```python
from build123d import *

# Parameters (mm, degrees)
SKETCH1_W                   = 203.2
SKETCH1_H                   = 203.2
BOSS_EXTRUDE1_DEPTH         = 6.35
CUT_EXTRUDE1_REACH          = 8.35
SKETCH2_R                   = 76.2
F_1_4_20_TAPPED_HOLE1_D     = 5.1054
F_1_4_20_TAPPED_HOLE1_DEPTH = 6.351
CIRPATTERN1_COUNT           = 12
CUT_EXTRUDE2_REACH          = 8.35


with BuildPart() as part:
    # Sketch1 → Boss-Extrude1 (new body)
    with BuildSketch(Plane(origin=(0, 0, 0), x_dir=(1, 0, 0), z_dir=(0, 1, 0))):
        Rectangle(SKETCH1_W, SKETCH1_H)
    extrude(amount=BOSS_EXTRUDE1_DEPTH)

    # Sketch2 → Cut-Extrude1 (cut, up to next)
    with BuildSketch(Plane(origin=(0, 6.35, 0), x_dir=(1, 0, 0), z_dir=(0, 1, 0)), mode=Mode.PRIVATE) as cut_extrude1_sk1:
        with Locations(Location((0, 0, 0), (0, 0, 270))):  # turned: the seam where the file's is
            Circle(SKETCH2_R)
    cut_extrude1_tool1 = extrude(cut_extrude1_sk1.sketch, amount=-CUT_EXTRUDE1_REACH, mode=Mode.PRIVATE) & part.part
    add(cut_extrude1_tool1.solids().sort_by_distance((0, 6.35, 0))[0], mode=Mode.SUBTRACT)

    # 1/4-20 Tapped Hole1
    with Locations(Plane(origin=(0, 6.35, 0), x_dir=(1, 0, 0), z_dir=(0, 1, 0))):
        with Locations((0, 85.725)):
            f_1_4_20_tapped_hole1 = Hole(F_1_4_20_TAPPED_HOLE1_D / 2, depth=F_1_4_20_TAPPED_HOLE1_DEPTH)

    # CirPattern1: 1/4-20 Tapped Hole1 ×12 about axis
    cirpattern1_axis = Axis((0, 0, 0), (0, 1, 0))
    for i in range(1, CIRPATTERN1_COUNT):
        add(f_1_4_20_tapped_hole1.rotate(cirpattern1_axis, i * 360 / CIRPATTERN1_COUNT), mode=Mode.SUBTRACT)

    # Sketch5 → Cut-Extrude2 (cut, up to next)
    with BuildSketch(Plane(origin=(0, 6.35, 0), x_dir=(1, 0, 0), z_dir=(0, 1, 0)), mode=Mode.PRIVATE) as cut_extrude2_sk1:
        with BuildLine():
            ThreePointArc((-45.084916162, 96.684914721), (-75.434151417, 75.434151417), (-96.684914721, 45.084916162))
            ThreePointArc((-96.684914721, 45.084916162), (-95.149200478, 40.865575958), (-90.929860273, 42.4012902))
            ThreePointArc((-90.929860273, 42.4012902), (-70.944023356, 70.944023356), (-42.4012902, 90.929860273))
            ThreePointArc((-42.4012902, 90.929860273), (-40.865575958, 95.149200478), (-45.084916162, 96.684914721))
        make_face()
    cut_extrude2_tool1 = extrude(cut_extrude2_sk1.sketch, amount=-CUT_EXTRUDE2_REACH, mode=Mode.PRIVATE) & part.part
    add(cut_extrude2_tool1.solids().sort_by_distance((-71.522214, 6.35, -71.522214))[0], mode=Mode.SUBTRACT)
    # Sketch5 → Cut-Extrude2 (cut, up to next)
    with BuildSketch(Plane(origin=(0, 6.35, 0), x_dir=(1, 0, 0), z_dir=(0, 1, 0)), mode=Mode.PRIVATE) as cut_extrude2_sk2:
        with BuildLine():
            ThreePointArc((96.684914721, 45.084916162), (75.434151417, 75.434151417), (45.084916162, 96.684914721))
            ThreePointArc((45.084916162, 96.684914721), (40.865575958, 95.149200478), (42.4012902, 90.929860273))
            ThreePointArc((42.4012902, 90.929860273), (70.944023356, 70.944023356), (90.929860273, 42.4012902))
            ThreePointArc((90.929860273, 42.4012902), (95.149200478, 40.865575958), (96.684914721, 45.084916162))
        make_face()
    cut_extrude2_tool2 = extrude(cut_extrude2_sk2.sketch, amount=-CUT_EXTRUDE2_REACH, mode=Mode.PRIVATE) & part.part
    add(cut_extrude2_tool2.solids().sort_by_distance((71.522214, 6.35, -71.522214))[0], mode=Mode.SUBTRACT)
    # Sketch5 → Cut-Extrude2 (cut, up to next)
    with BuildSketch(Plane(origin=(0, 6.35, 0), x_dir=(1, 0, 0), z_dir=(0, 1, 0)), mode=Mode.PRIVATE) as cut_extrude2_sk3:
        with BuildLine():
            ThreePointArc((-96.684914721, -45.084916162), (-75.434151417, -75.434151417), (-45.084916162, -96.684914721))
            ThreePointArc((-45.084916162, -96.684914721), (-40.865575958, -95.149200478), (-42.4012902, -90.929860273))
            ThreePointArc((-42.4012902, -90.929860273), (-70.944023356, -70.944023356), (-90.929860273, -42.4012902))
            ThreePointArc((-90.929860273, -42.4012902), (-95.149200478, -40.865575958), (-96.684914721, -45.084916162))
        make_face()
    cut_extrude2_tool3 = extrude(cut_extrude2_sk3.sketch, amount=-CUT_EXTRUDE2_REACH, mode=Mode.PRIVATE) & part.part
    add(cut_extrude2_tool3.solids().sort_by_distance((-71.522214, 6.35, 71.522214))[0], mode=Mode.SUBTRACT)
    # Sketch5 → Cut-Extrude2 (cut, up to next)
    with BuildSketch(Plane(origin=(0, 6.35, 0), x_dir=(1, 0, 0), z_dir=(0, 1, 0)), mode=Mode.PRIVATE) as cut_extrude2_sk4:
        with BuildLine():
            ThreePointArc((45.084916162, -96.684914721), (75.434151417, -75.434151417), (96.684914721, -45.084916162))
            ThreePointArc((96.684914721, -45.084916162), (95.149200478, -40.865575958), (90.929860273, -42.4012902))
            ThreePointArc((90.929860273, -42.4012902), (70.944023356, -70.944023356), (42.4012902, -90.929860273))
            ThreePointArc((42.4012902, -90.929860273), (40.865575958, -95.149200478), (45.084916162, -96.684914721))
        make_face()
    cut_extrude2_tool4 = extrude(cut_extrude2_sk4.sketch, amount=-CUT_EXTRUDE2_REACH, mode=Mode.PRIVATE) & part.part
    add(cut_extrude2_tool4.solids().sort_by_distance((71.522214, 6.35, 71.522214))[0], mode=Mode.SUBTRACT)


solid = part.part
```
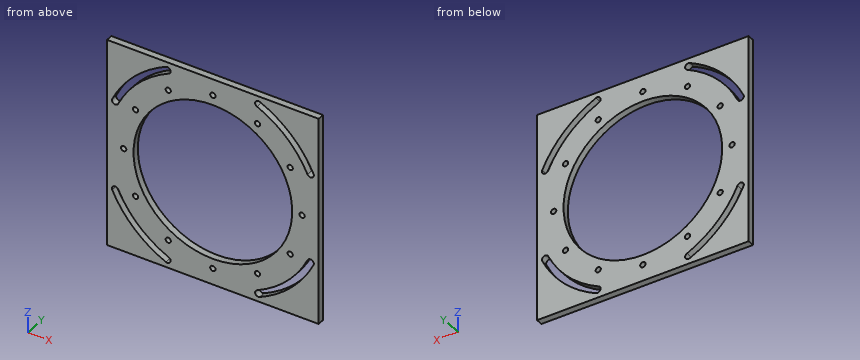
Verification items for the finished model (mm, model axes). Coordinates: 2 decimals unless noted, no trailing zeros. Write each loop counter-clockwise with the first axis right and the second up, starting at its lowest first coordinate (ties: lowest second). Pieces come first, ordered by that corner, then holes. Notation, with made-up numbers: M 36,14.25 L 82,14.25 A14 cw 82,19.25 Z; hole C 0.5,78.5 d10. An arc over 180 degrees is marked long. Answer as a JSON object with one key per item and string values. Group by question number.
(1) Cross-section at D-D, the plane y = 2.25. State how many separate pieces and enclosed holes the cut face has, and give its area (3 significant figures).
(2) Gauge pin test, flat end, axial feed: pin 1 (1 mm diameter, centred on x = -35.5, z = -66.5, fed in from -Y). Record the tip position at first contact, or that the pin passes through.
(3) Material ranges on line 1 (X direction, y = 0.5, z = -83); line 2 (Z direction, x = 56, y = 4.5); line 3 (Z direction, x = -64, y = 5), recorded low to high.
(4) Cross-section at A-A, the plane z = 0. Record the cut outline in (x, y).
(5) Cross-section at B-B, the plane x = 0. Record the cut outline in (y, z), and give its area (3 significant figures).
(6) Cross-section at C-C, the plane z = 22. Record the cut outline in (x, y).
Reply:
{
 "1": {"separate pieces": "1", "enclosed holes": "17", "area": "20,800 mm²"},
 "2": {"pin 1": "through"},
 "3": {"line 1": "-101.6 to -67.02, -56.37 to 56.37, 67.02 to 101.6", "line 2": "-101.6 to -90.8, -83.25 to -51.68, 51.68 to 83.25, 90.8 to 101.6", "line 3": "-101.6 to -85.35, -77.27 to -41.36, 41.36 to 77.27, 85.35 to 101.6"},
 "4": {"outline": "M -101.6,0 L -88.28,0 L -88.28,6.35 L -101.6,6.35 Z; M -83.17,0 L -76.2,0 L -76.2,6.35 L -83.17,6.35 Z; M 76.2,0 L 83.17,0 L 83.17,6.35 L 76.2,6.35 Z; M 88.28,0 L 101.6,0 L 101.6,6.35 L 88.28,6.35 Z"},
 "5": {"outline": "M 0,-101.6 L 6.35,-101.6 L 6.35,-88.28 L 0,-88.28 Z; M 0,-83.17 L 6.35,-83.17 L 6.35,-76.2 L 0,-76.2 Z; M 0,76.2 L 6.35,76.2 L 6.35,83.17 L 0,83.17 Z; M 0,88.28 L 6.35,88.28 L 6.35,101.6 L 0,101.6 Z", "area": "258 mm²"},
 "6": {"outline": "M -101.6,0 L -72.96,0 L -72.96,6.35 L -101.6,6.35 Z; M 72.96,0 L 101.6,0 L 101.6,6.35 L 72.96,6.35 Z"}
}
